from build123d import *

# Parameters (mm, degrees)
F0_W     = 120.965316
F0_H     = 76.2
F0_R     = 1.7272
F0_W_2   = 11.536045
F0_H_2   = 24
F0_R_2   = 2.15265
F1_DEPTH = 3.175


with BuildPart() as f1:
    # F0 (on Top) → F1 (new body)
    with BuildSketch(Plane.XY):
        Rectangle(F0_W, F0_H)
        with Locations((-35.36249, -33.3375)):
            Circle(F0_R, mode=Mode.SUBTRACT)
        with Locations((-50.8, -22.925)):
            Rectangle(F0_W_2, F0_H_2, mode=Mode.SUBTRACT)
        with Locations((35.36249, -33.3375)):
            Circle(F0_R, mode=Mode.SUBTRACT)
        with Locations((50.8, -22.925)):
            Rectangle(F0_W_2, F0_H_2, mode=Mode.SUBTRACT)
        with Locations((-7.14375, 0)):
            Circle(F0_R_2, mode=Mode.SUBTRACT)
        with Locations((-50.8, 22.925)):
            Rectangle(F0_W_2, F0_H_2, mode=Mode.SUBTRACT)
        with Locations((-35.36249, 33.3375)):
            Circle(F0_R, mode=Mode.SUBTRACT)
        with Locations((7.14375, 0)):
            Circle(F0_R_2, mode=Mode.SUBTRACT)
        Polygon((45.031977, 34.925), (56.568022, 34.925), (56.568023, 10.925), (45.031978, 10.925), align=None, mode=Mode.SUBTRACT)
        with Locations((35.36249, 33.3375)):
            Circle(F0_R, mode=Mode.SUBTRACT)
    extrude(amount=F1_DEPTH)


solid = f1.part
Geometry check sheet. Reference: the model listing, model coordinates, mm. A direction names the side the tool comes from. Coordinates: 2 decimals unless noted, no trailing zeros. Order: outer loops, then holes, each group sorted by start corner. A loop starts at its lowest first (then second) coordinate and runs counter-clockwise, first axis right, second up. Notation, with made-up numbers: (-23.75, 58) -> (-19.75, 58) arc R22 ccw to (-19.75, 79) -> close; hole circle Ø9 at (-19.5, 3). An arc over 180 degrees is marked (long way). Use a Markdown table: item, result. Add a question column.
1. Cross-section at C-C (y = -14.5). Enter the section's corners in (x, z) (3 decimals), and give its area (3 significant figures).
2. Material ranges on L1, parallel to X at y = 24.5, z = 0.8; L2, parallel to Y at x = -47, z = 2.05 (3 decimals); L3, parallel to Y at x = -35, z = 2.5, recorded low to high.
3. Cross-section at A-A (y = 0). Enter the section's corners in (x, z) (3 decimals), and give its area (3 significant figures).
4. Set-up check for faces 5 (the face through (-56.568, -23, 2)), 6 (the face through (-1, 38.1, 2)): record each of +Z, -Z, +X, -X, +Y, -Y from which the full face is reachable in a straight line by a thin tool's end or side.
5. Mould release check, pull along X, two halves, no side actions. Record for faces 1 (the face through (-60.483, -1, 2)), 2 (the face through (-1, 1, 3.175)), 3 (the face through (56.568, -23, 2)), 4 (the face through (-45.032, -23, 2)): pulls with the +X half, pulls with the -X half, needs draft (parallel to the pull), parting line crosses it, or undercut.
6. Cross-section at B-B (x = 6.5). Enter the section's corners in (y, z) (3 decimals), and give its area (3 significant figures).
7. Cross-section at D-D (z = 0.6). Give the number of separate pieces and of enclosed holes in the cut face, and give its area (3 significant figures).
8. Go/stop test with a flat-tipped pin: pin 1 Ø3 at (x, y) = (-35.36, 33.34) entering from +Z. Record where the tip stops, or that it passes through.
Filled sheet:
| question | item | result |
|---|---|---|
| 1 | outline | (-60.483, 0) -> (-56.568, 0) -> (-56.568, 3.175) -> (-60.483, 3.175) -> close; (-45.032, 0) -> (45.032, 0) -> (45.032, 3.175) -> (-45.032, 3.175) -> close; (56.568, 0) -> (60.483, 0) -> (60.483, 3.175) -> (56.568, 3.175) -> close |
| 1 | area | 311 mm2 |
| 2 | L1 | -60.48 to -56.57, -45.03 to 45.03, 56.57 to 60.48 |
| 2 | L2 | -38.1 to -34.925, -10.925 to 10.925, 34.925 to 38.1 |
| 2 | L3 | -38.1 to -35.03, -31.65 to 31.65, 35.03 to 38.1 |
| 3 | outline | (-60.483, 0) -> (-9.296, 0) -> (-9.296, 3.175) -> (-60.483, 3.175) -> close; (-4.991, 0) -> (4.991, 0) -> (4.991, 3.175) -> (-4.991, 3.175) -> close; (9.296, 0) -> (60.483, 0) -> (60.483, 3.175) -> (9.296, 3.175) -> close |
| 3 | area | 357 mm2 |
| 4 | face 5 | +Z, -Z |
| 4 | face 6 | +Z, -Z, +X, -X, +Y |
| 5 | face 1 | pulls with the -X half |
| 5 | face 2 | needs draft |
| 5 | face 3 | undercut |
| 5 | face 4 | undercut |
| 6 | outline | (-38.1, 0) -> (-2.054, 0) -> (-2.054, 3.175) -> (-38.1, 3.175) -> close; (2.054, 0) -> (38.1, 0) -> (38.1, 3.175) -> (2.054, 3.175) -> close |
| 6 | area | 229 mm2 |
| 7 | separate pieces | 1 |
| 7 | enclosed holes | 10 |
| 7 | area | 8,040 mm2 |
| 8 | pin 1 | through |
